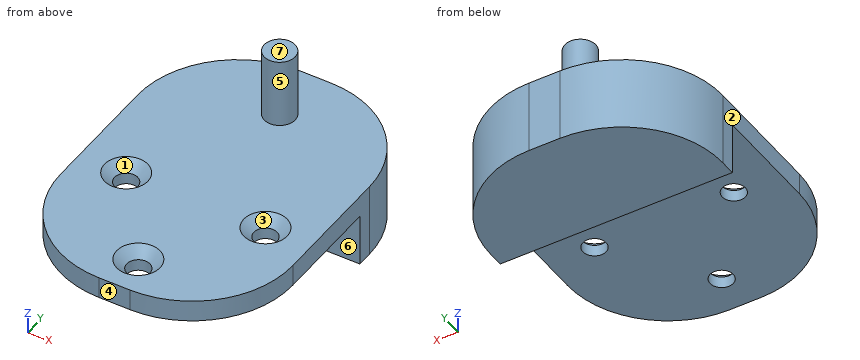
from build123d import *

# Parameters (mm, degrees)
F0_W           = 27
F0_H           = 2.8
F1_DEPTH       = 15
F2_R           = 13
F3_R           = 13
F5_D           = 3
F5_CSINK_D     = 5.6
F5_CSINK_ANGLE = 90
F6_D           = 3
F6_CSINK_D     = 5.6
F6_CSINK_ANGLE = 90
F7_D           = 3
F7_CSINK_D     = 5.6
F7_CSINK_ANGLE = 90
F8_R           = 2
F9_DEPTH       = 9


with BuildPart() as f1:
    # F0 (on Right) → F1 (new body, symmetric)
    with BuildSketch(Plane.YZ):
        Polygon((15, 1.068751), (0, 1.068751), (0, -1.731249), (0, -8.531249), (15, -8.531249), align=None)
        with Locations((-13.5, -0.331249)):
            Rectangle(F0_W, F0_H)
    extrude(amount=F1_DEPTH, both=True)

    # F2
    f2_edges = [f1.edges().sort_by_distance(p)[0] for p in [
        (15, 15, -3.731249),
        (-15, 15, -3.731249),
    ]]
    fillet(f2_edges, radius=F2_R)

    # F3
    f3_edges = [f1.edges().sort_by_distance(p)[0] for p in [
        (15, -27, -0.331249),
        (-15, -27, -0.331249),
    ]]
    fillet(f3_edges, radius=F3_R)

    # F5 (through all)
    with Locations(Plane.XY.offset(1.068751)):
        with Locations((-9, -10)):
            CounterSinkHole(F5_D / 2, F5_CSINK_D / 2, counter_sink_angle=F5_CSINK_ANGLE)

    # F6 (through all)
    with Locations(Plane.XY.offset(1.068751)):
        with Locations((9, -10)):
            CounterSinkHole(F6_D / 2, F6_CSINK_D / 2, counter_sink_angle=F6_CSINK_ANGLE)

    # F7 (through all)
    with Locations(Plane.XY.offset(1.068751)):
        with Locations((0, -22)):
            CounterSinkHole(F7_D / 2, F7_CSINK_D / 2, counter_sink_angle=F7_CSINK_ANGLE)

    # F8 (on face) → F9 (join, symmetric)
    with BuildSketch(Plane.XY.offset(1.068751)):
        with Locations((0, 7.5)):
            Circle(F8_R)
    extrude(amount=F9_DEPTH, both=True)


solid = f1.part
Here's how the part is built. I have some questions about the finished solid (model axes, mm). Face numbers are marked on the shaded views. A direction names the side the tool comes from. Round coordinates to 2 decimals unless told otherwise and drop trailing zeros. Loops run counter-clockwise (first coordinate to the right, second up) from the corner with the lowest first, then second, coordinate; pieces in that order, holes last. Notation, with made-up numbers: (17, 58) - (30, 58) arc R26 ccw to (30, 87) - close; hole circle Ø7 at (-39, -1.75). An arc over 180 degrees is marked (long way). One line per question, with ' | ' between items. Start each with the question number.
Q1. Please list where these lines run through material, in increasing order: line 1 (X direction, y = -10, z = -1.15); line 2 (Z direction, x = -4.5, y = -17.5); line 3 (Z direction, x = 3, y = 5). Write a range as [from, to].
Q2. I want a section at C-C (z = -3.75). Write out the boundary of the cut face in (x, y), then the cut area to 3 significant figures.
Q3. We'd pull the mould along Y, two halves only. Please class the marked faces 1, 2, 3 and 4: +Y half, -Y half, draft (parallel to the pull), parting line (faces both ways), or undercut.
Q4. I want a section at B-B (x = 0). Write out the boundary of the cut face in (y, z), then the cut area to 3 significant figures.
Q5. Will these pins go through, and if not, where does the flat tip stop? pin 1 (6 mm diameter, centred on y = 9, z = 4.5, fed in from +X); pin 2 (3.5 mm diameter, centred on x = 6, z = -7, fed in from -Y); pin 3 (5 mm diameter, centred on x = 9, y = -10, fed in from +Z).
Q6. For the marked faces 5, 6 and 7, which set-ups out of +Z, -Z, +X, -X, +Y, -Y let a thin tool reach every point of the face, with its end or its side?
Q7. I want a section at A-A (y = -10). Write out the boundary of the cut face in (x, z).
Q8. I want a section at D-D (z = 0.25). Write out the boundary of the cut face in (x, y), then the cut area to 3 significant figures.
Response values:
1) line 1: x = [-15, -10.5], [-7.5, 7.5], [10.5, 15] | line 2: z = [-1.73, 1.07] | line 3: z = [-8.53, 1.07]
2) outline: (-15, 0) - (15, 0) - (15, 2) arc R13 ccw to (2, 15) - (-2, 15) arc R13 ccw to (-15, 2) - close | area: 377 mm²
3) face 1: undercut | face 2: draft | face 3: undercut | face 4: -Y half
4) outline: (-27, -1.73) - (-23.5, -1.73) - (-23.5, -0.23) - (-24.8, 1.07) - (-27, 1.07) - close; (-20.5, -1.73) - (0, -1.73) - (0, -8.53) - (15, -8.53) - (15, 1.07) - (9.5, 1.07) - (9.5, 10.07) - (5.5, 10.07) - (5.5, 1.07) - (-19.2, 1.07) - (-20.5, -0.23) - close | area: 246 mm²
5) pin 1: stops at x = 2 | pin 2: stops at y = 0 | pin 3: stops at z = 0.77
6) face 5: +Z | face 6: -Z, +X, -X, -Y | face 7: +Z, +X, -X, +Y, -Y
7) outline: (-15, -1.73) - (-10.5, -1.73) - (-10.5, -0.23) - (-11.8, 1.07) - (-15, 1.07) - close; (-7.5, -1.73) - (7.5, -1.73) - (7.5, -0.23) - (6.2, 1.07) - (-6.2, 1.07) - (-7.5, -0.23) - close; (10.5, -1.73) - (15, -1.73) - (15, 1.07) - (11.8, 1.07) - (10.5, -0.23) - close
8) outline: (-15, -14) arc R13 ccw to (-2, -27) - (2, -27) arc R13 ccw to (15, -14) - (15, 2) arc R13 ccw to (2, 15) - (-2, 15) arc R13 ccw to (-15, 2) - close; hole circle Ø3.96 at (-9, -10); hole circle Ø3.96 at (0, -22); hole circle Ø3.96 at (9, -10) | area: 1,080 mm²
